Verification items for the finished model (mm, model axes). Face numbers are marked on the shaded views. A direction names the side the tool comes from. Round coordinates to 2 decimals unless told otherwise and drop trailing zeros. Loops run counter-clockwise (first coordinate to the right, second up) from the corner with the lowest first, then second, coordinate; pieces in that order, holes last. Notation, with made-up numbers: M 84,65 L 112,65 A24 cw 112,104 Z; hole C 1,-10.5 d2. An arc over 180 degrees is marked long. Answer as CSV lines item,"result".
```python
from build123d import *

# Parameters (mm, degrees)
SKETCH1_W                  = 72
SKETCH1_H                  = 7
BOSS_EXTRUDE1_DEPTH        = 55
BOSS_EXTRUDE2_DEPTH        = 7
BOSS_EXTRUDE3_DEPTH        = 39
BOSS_EXTRUDE4_START        = 7.5
BOSS_EXTRUDE4_DEPTH        = 24
FILLET1_RADIUS             = 12
FILLET1_LENGTH             = 7
FILLET2_RADIUS             = 12
FILLET2_LENGTH             = 7
F_1_0MM_DOWEL_HOLE1_D      = 15
RIB1_REACH                 = 119.589
SKETCH4_WALL_W             = 272.06418258
SKETCH4_WALL_H             = 8
FILLET3_R                  = 16
F_12_0MM_DOWEL_HOLE1_D     = 12
F_12_0MM_DOWEL_HOLE1_DEPTH = 7


with BuildPart() as part:
    # Sketch1 → Boss-Extrude1 (new body)
    with BuildSketch(Plane.XY):
        Rectangle(SKETCH1_W, SKETCH1_H)
    extrude(amount=BOSS_EXTRUDE1_DEPTH)

    # Sketch1<3> → Boss-Extrude2 (add)
    with BuildSketch(Plane.XY):
        with BuildLine():
            ThreePointArc((19, 53.5), (-2.93819909, 34.728559296), (-18.091261695, 59.305708421))
            Line((-18.091261695, 59.305708421), (-36, 3.5))
            Line((-36, 3.5), (36, 3.5))
            Line((36, 3.5), (18.091261695, 59.305708421))
            ThreePointArc((18.091261695, 59.305708421), (18.771440704, 56.43819909), (19, 53.5))
        make_face()
    extrude(amount=BOSS_EXTRUDE2_DEPTH)

    # Sketch1<4> → Boss-Extrude3 (add)
    with BuildSketch(Plane.XY):
        with BuildLine():
            ThreePointArc((-8.5, 70.492645468), (-14.424308987, 65.866863395), (-18.091261695, 59.305708421))
            ThreePointArc((-18.091261695, 59.305708421), (-2.93819909, 34.728559296), (19, 53.5))
            ThreePointArc((19, 53.5), (18.771440704, 56.43819909), (18.091261695, 59.305708421))
            ThreePointArc((18.091261695, 59.305708421), (14.424308987, 65.866863395), (8.5, 70.492645468))
            ThreePointArc((8.5, 70.492645468), (5.093989215, 71.80440586), (1.5, 72.440696925))
            Line((1.5, 72.440696925), (1.5, 65.4058809))
            ThreePointArc((1.5, 65.4058809), (9, 61.437253933), (12, 53.5))
            ThreePointArc((12, 53.5), (-7.937253933, 44.5), (-1.5, 65.4058809))
            Line((-1.5, 65.4058809), (-1.5, 72.440696925))
            ThreePointArc((-1.5, 72.440696925), (-5.093989215, 71.80440586), (-8.5, 70.492645468))
        make_face()
    extrude(amount=BOSS_EXTRUDE3_DEPTH)

    # Sketch1<5> → Boss-Extrude4 (add)
    with BuildSketch(Plane.XY.offset(BOSS_EXTRUDE4_START)):
        with BuildLine():
            Line((1.5, 97.5), (1.5, 72.440696925))
            ThreePointArc((1.5, 72.440696925), (5.093989215, 71.80440586), (8.5, 70.492645468))
            Line((8.5, 70.492645468), (8.5, 97.5))
            Line((8.5, 97.5), (1.5, 97.5))
        make_face()
        with BuildLine():
            Line((-8.5, 97.5), (-8.5, 70.492645468))
            ThreePointArc((-8.5, 70.492645468), (-5.093989215, 71.80440586), (-1.5, 72.440696925))
            Line((-1.5, 72.440696925), (-1.5, 97.5))
            Line((-1.5, 97.5), (-8.5, 97.5))
        make_face()
    extrude(amount=BOSS_EXTRUDE4_DEPTH)

    # Fillet1: full round fillet: the end face becomes a half cylinder, R = half its width
    fillet1_face = Plane((5, 97.5, 19.5), x_dir=(1, 0, 0), z_dir=(0, 1, 0))  # on the end face: x along it, z out of the body
    fillet1_slab = fillet1_face.offset(-FILLET1_RADIUS / 2) * Box(FILLET1_LENGTH, 2 * FILLET1_RADIUS, FILLET1_RADIUS, mode=Mode.PRIVATE)  # the body's end, R deep
    fillet1_round = Plane((5, 85.5, 19.5), x_dir=(0, 1, 0), z_dir=(1, 0, 0)) * Cylinder(FILLET1_RADIUS, FILLET1_LENGTH, mode=Mode.PRIVATE)  # its axis R under the face
    add(fillet1_slab - fillet1_round, mode=Mode.SUBTRACT)

    # Fillet2: full round fillet: the end face becomes a half cylinder, R = half its width
    fillet2_face = Plane((-5, 97.5, 19.5), x_dir=(-1, 0, 0), z_dir=(0, 1, 0))  # on the end face: x along it, z out of the body
    fillet2_slab = fillet2_face.offset(-FILLET2_RADIUS / 2) * Box(FILLET2_LENGTH, 2 * FILLET2_RADIUS, FILLET2_RADIUS, mode=Mode.PRIVATE)  # the body's end, R deep
    fillet2_round = Plane((-5, 85.5, 19.5), x_dir=(0, 1, 0), z_dir=(-1, 0, 0)) * Cylinder(FILLET2_RADIUS, FILLET2_LENGTH, mode=Mode.PRIVATE)  # its axis R under the face
    add(fillet2_slab - fillet2_round, mode=Mode.SUBTRACT)

    # Ø1.0mm Dowel Hole1 (through all)
    with Locations(Plane(origin=(8.5, 0, 0), x_dir=(0, 0, -1), z_dir=(1, 0, 0))):
        with Locations((-19.5, 85.5)):
            Hole(F_1_0MM_DOWEL_HOLE1_D / 2)

    # Sketch4 wall → Rib1 (add, up to next)
    with BuildSketch(Plane(origin=(0, 19, 47), x_dir=(0, -0.888620657055, 0.45864291977), z_dir=(0, -0.45864291977, -0.888620657055)), mode=Mode.PRIVATE) as rib1_sk1:
        Rectangle(SKETCH4_WALL_W, SKETCH4_WALL_H)
    rib1_tool1 = extrude(rib1_sk1.sketch, amount=RIB1_REACH, mode=Mode.PRIVATE) - part.part
    add(rib1_tool1.solids().sort_by_distance((0, 19, 47))[0])

    # Fillet3
    fillet3_edges = [part.edges().sort_by_distance(p)[0] for p in [
        (36, 0, 55),
        (-36, 0, 55),
    ]]
    fillet(fillet3_edges, radius=FILLET3_R)

    # Ø12.0mm Dowel Hole1
    with Locations(Plane(origin=(0, 3.5, 0), x_dir=(1, 0, 0), z_dir=(0, 1, 0))):
        with Locations((20, -39), (-20, -39)):
            Hole(F_12_0MM_DOWEL_HOLE1_D / 2, depth=F_12_0MM_DOWEL_HOLE1_DEPTH)


solid = part.part
```
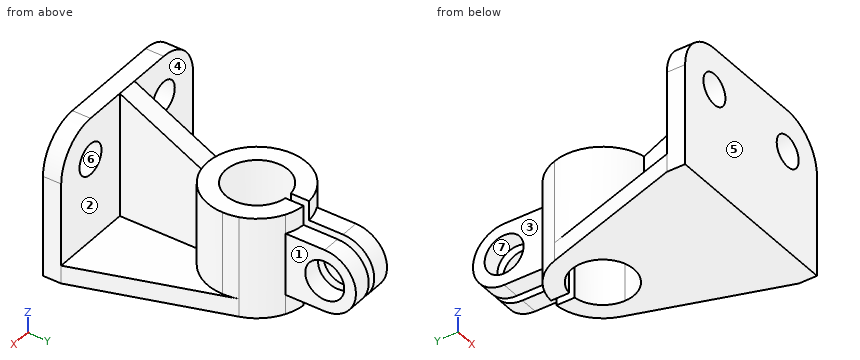
1) Section check D-D (y = 38). Record the cut outline in (x, z).
Here are the results:
outline,"M -24.93,0 L 24.93,0 L 24.93,7 L 10.99,7 L 10.99,39 L -10.99,39 L -10.99,7 L -24.93,7 Z"
2) Go/stop test with flat-tipped pins: pin 1 (1 mm diameter, centred on y = 15.5, z = 8, fed in from +X); pin 2 (10 mm diameter, centred on y = 33, z = 20, fed in from -X); pin 3 (9.5 mm diameter, centred on x = 24.5, y = 28.5, fed in from +Z); pin 4 (2 mm diameter, centred on y = 31, z = 44, fed in from -X). Record where each tip stops, or that it passes through.
Here are the results:
pin 1,"stops at x = 4"
pin 2,"stops at x = -10.99"
pin 3,"stops at z = 7"
pin 4,"passes through"
3) Section check A-A (z = 19.5). Record the cut outline in (x, y), plus the area to 3 significant figures.
Here are the results:
outline,"M -36,-3.5 L 36,-3.5 L 36,3.5 L 4,3.5 L 4,34.93 A19 ccw 8.5,70.49 L 8.5,78 L 1.5,78 L 1.5,65.41 A12 cw long -1.5,65.41 L -1.5,78 L -8.5,78 L -8.5,70.49 A19 ccw -4,34.93 L -4,3.5 L -36,3.5 Z; M -8.5,93 L -1.5,93 L -1.5,97.5 L -8.5,97.5 Z; M 1.5,93 L 8.5,93 L 8.5,97.5 L 1.5,97.5 Z"
area,"1,560 mm^2"
4) Section check B-B (y = 75.5). Record the cut outline in (x, z), plus the area to 3 significant figures.
Here are the results:
outline,"M -8.5,7.5 L -1.5,7.5 L -1.5,31.5 L -8.5,31.5 Z; M 1.5,7.5 L 8.5,7.5 L 8.5,31.5 L 1.5,31.5 Z"
area,"336 mm^2"
5) Material ranges on probe 1 along X at (y, z) = (-1, 39); probe 2 along Y at (x, z) = (8, 35.5); probe 3 along X at (y, z) = (53, 29), recorded low to high.
Here are the results:
probe 1,"x = -36 to -26, -14 to 14, 26 to 36"
probe 2,"y = -3.5 to 3.5, 36.27 to 44.56, 62.44 to 70.73"
probe 3,"x = -18.99 to -11.99, 11.99 to 18.99"
6) Draft check along Y on the marked faces 5, 6 and 7. Enter one of: +Y half, -Y half, draft (parallel to the pull), parting line (faces both ways), or undercut.
Here are the results:
face 5,"-Y half"
face 6,"draft"
face 7,"undercut"
7) Set-up check for the marked faces 1, 2, 3 and 4: record each of +Z, -Z, +X, -X, +Y, -Y from which the full face is reachable in a straight line by a thin tool's end or side.
Here are the results:
face 1,"+Z, -Z, +X, +Y"
face 2,"+Z, +X"
face 3,"+Z, -Z, -X, +Y"
face 4,"+Z, -X"
8) Section check C-C (z = 3.5). Record the cut outline in (x, y), plus the area to 3 significant figures.
Here are the results:
outline,"M -36,-3.5 L 36,-3.5 L 36,3.5 L 18.09,59.31 A19 ccw 1.5,72.44 L 1.5,65.41 A12 cw long -1.5,65.41 L -1.5,72.44 A19 ccw -18.09,59.31 L -36,3.5 Z"
area,"3,400 mm^2"
